Part model, mm, in its own coordinate system. Give positions to 0.01 mm unless a question says otherwise; leave off trailing zeros. Write each loop counter-clockwise with the first axis right and the second up, starting at its lowest first coordinate (ties: lowest second). Pieces come first, ordered by that corner, then holes. Notation, with made-up numbers: (56.25, 69) - (62.25, 69) arc R21 ccw to (62.25, 90) - close; hole circle Ø10 at (-37, 68). An arc over 180 degrees is marked (long way). Answer as a JSON object with one key per item and string values. Group by question number.
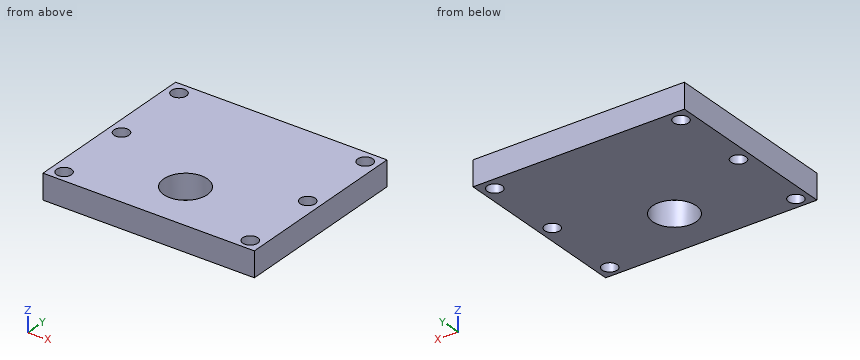
```python
from build123d import *

# Parameters (mm, degrees)
SKETCH1_W                 = 53.34
SKETCH1_H                 = 45.72
BOSS_EXTRUDE1_DEPTH       = 6.35
SKETCH2_R                 = 5.5
CUT_EXTRUDE1_DEPTH        = 1
CUT_EXTRUDE1_DEPTH_BACK   = 7.35
F_6_CLEARANCE_HOLE1_D     = 3.7973
F_6_CLEARANCE_HOLE1_DEPTH = 6.35


with BuildPart() as part:
    # Sketch1 → Boss-Extrude1 (new body)
    with BuildSketch(Plane.XY):
        with Locations((26.67, 22.86)):
            Rectangle(SKETCH1_W, SKETCH1_H)
    extrude(amount=BOSS_EXTRUDE1_DEPTH)

    # Sketch2 → Cut-Extrude1 (cut, two sides)
    with BuildSketch(Plane.XY.offset(6.35)) as cut_extrude1_sk:
        with Locations((26.67, 12.7)):
            Circle(SKETCH2_R)
    extrude(amount=CUT_EXTRUDE1_DEPTH, mode=Mode.SUBTRACT)
    extrude(cut_extrude1_sk.sketch, amount=-CUT_EXTRUDE1_DEPTH_BACK, mode=Mode.SUBTRACT)

    # #6 Clearance Hole1
    with Locations(Plane.XY.offset(6.35)):
        with Locations((3.175, 42.545), (50.165, 42.545), (50.165, 22.733), (50.165, 2.921), (3.175, 22.733), (3.175, 2.921)):
            Hole(F_6_CLEARANCE_HOLE1_D / 2, depth=F_6_CLEARANCE_HOLE1_DEPTH)


solid = part.part
```
1) Drill centre lines: line 1 along X through (y, z) = (24, 5.5); line 2 along X through (y, z) = (13.5, 5.25); line 3 along Y through (x, z) = (28, 2.5). Where is each one in solid material? Low to high. Write a range as from..to.
2) Drop flat-ended pins along their axis: P1, Ø2, axis at y = 25.5, z = 3.5, coming from the -X side; P2, Ø3, axis at x = 50.165, y = 22.733, coming from the -Z side. Give the stop position or say it passes through.
3) Saw through at B-B (y = 12.7). List the corners of the cut face in (x, z), and give its area (3 significant figures).
4) Saw through at C-C (z = 3.5). List the corners of the cut face in (x, y) (3 decimals), and give its area (3 significant figures).
5) Saw through at A-A (x = 26.67). List the corners of the cut face in (y, z), and give its area (3 significant figures).
Checks:
{
 "1": {"line 1": "0..1.76, 4.59..48.75, 51.58..53.34", "line 2": "0..21.23, 32.11..53.34", "line 3": "0..7.36, 18.04..45.72"},
 "2": {"P1": "x = 0", "P2": "through"},
 "3": {"outline": "(0, 0) - (21.17, 0) - (21.17, 6.35) - (0, 6.35) - close; (32.17, 0) - (53.34, 0) - (53.34, 6.35) - (32.17, 6.35) - close", "area": "269 mm2"},
 "4": {"outline": "(0, 0) - (53.34, 0) - (53.34, 45.72) - (0, 45.72) - close; hole circle Ø3.797 at (3.175, 2.921); hole circle Ø3.797 at (3.175, 22.733); hole circle Ø3.797 at (3.175, 42.545); hole circle Ø11 at (26.67, 12.7); hole circle Ø3.797 at (50.165, 2.921); hole circle Ø3.797 at (50.165, 22.733); hole circle Ø3.797 at (50.165, 42.545)", "area": "2,280 mm2"},
 "5": {"outline": "(0, 0) - (7.2, 0) - (7.2, 6.35) - (0, 6.35) - close; (18.2, 0) - (45.72, 0) - (45.72, 6.35) - (18.2, 6.35) - close", "area": "220 mm2"}
}
